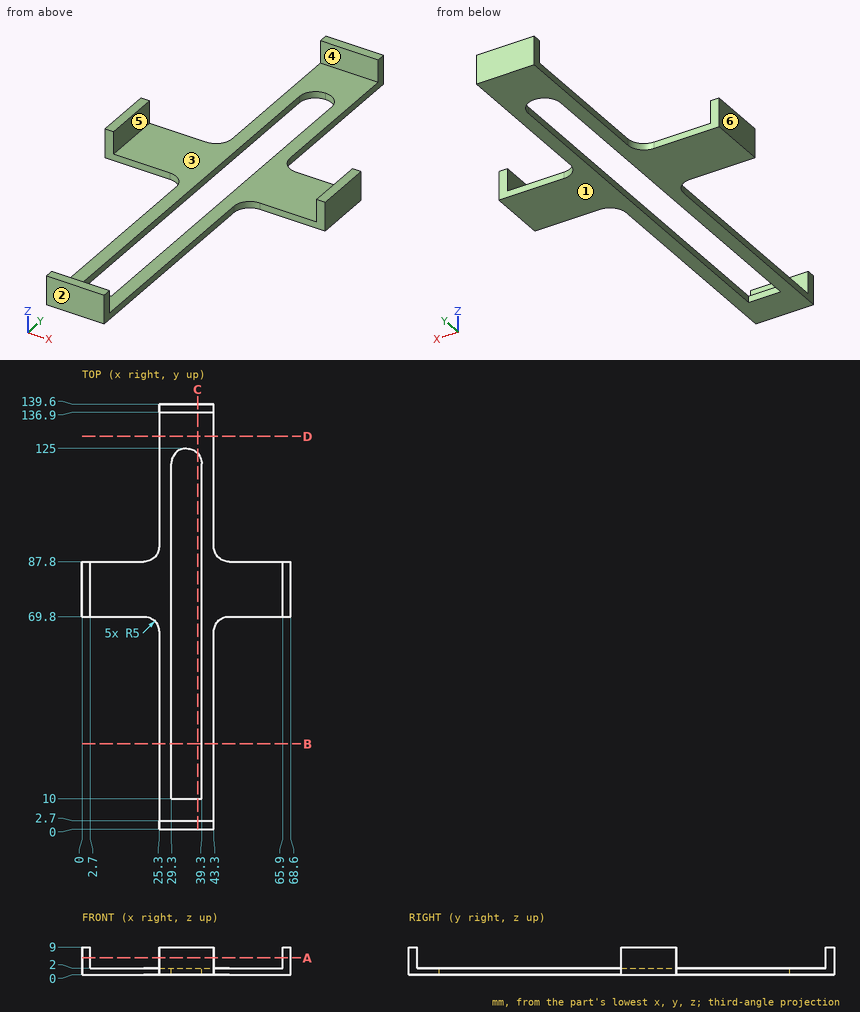
Verification items for this drawing (mm, ordinates from the low corner). A direction names the side the tool comes from. Round coordinates to 2 decimals unless told otherwise and drop trailing zeros. Write each loop counter-clockwise with the first axis right and the second up, starting at its lowest first coordinate (ties: lowest second). Pieces come first, ordered by that corner, then holes. Notation, with made-up numbers: (-8.75, 10) - (20.25, 10) arc R27 ccw to (20.25, 26) - close; hole circle Ø7 at (30.5, 26). An arc over 180 degrees is marked (long way). One line per item, written item: value.
1. Cross-section at C-C on x = 38. Record the boundary of the cut face in (y, z), and give its area (3 significant figures).
The answers:
outline: (0, 0) - (10, 0) - (10, 2) - (2.7, 2) - (2.7, 9) - (0, 9) - close; (123.36, 0) - (139.6, 0) - (139.6, 9) - (136.9, 9) - (136.9, 2) - (123.36, 2) - close
area: 90.3 mm^2
2. Cross-section at A-A on z = 5.5. Record the boundary of the cut face in (x, y).
The answers:
outline: (0, 69.8) - (2.7, 69.8) - (2.7, 87.8) - (0, 87.8) - close; (25.3, 0) - (43.3, 0) - (43.3, 2.7) - (25.3, 2.7) - close; (25.3, 136.9) - (43.3, 136.9) - (43.3, 139.6) - (25.3, 139.6) - close; (65.9, 69.8) - (68.6, 69.8) - (68.6, 87.8) - (65.9, 87.8) - close
3. Cross-section at D-D on y = 129. Record the boundary of the cut face in (x, z), and give its area (3 significant figures).
The answers:
outline: (25.3, 0) - (43.3, 0) - (43.3, 2) - (25.3, 2) - close
area: 36.0 mm^2
4. Depth check by flat-ended pin: pin 1 Ø5 at (x, z) = (50.5, 2) entering from -Y; pin 2 Ø3.5 at (x, z) = (33.5, 4) entering from -Y; pin 3 Ø2 at (y, z) = (64.5, 0.5) entering from -X; pin 4 Ø4 at (y, z) = (97.5, 3.5) entering from +X. Enter the tip coordinate at first touch or a pass-through.
The answers:
pin 1: stops at y = 69.79
pin 2: stops at y = 0
pin 3: stops at x = 25.25
pin 4: stops at x = 43.3
5. Set-up check for the marked faces 5 and 6: record each of +Z, -Z, +X, -X, +Y, -Y from which the full face is reachable in a straight line by a thin tool's end or side.
The answers:
face 5: +Z, +Y, -Y
face 6: +Z, -Z, -X, +Y, -Y
6. Mould release check, pull along Y, two halves, no side actions. Record for the marked faces 1, 2, 3 and 4: released by +Y, released by -Y, zero draft, split by the parting line, or undercut.
The answers:
face 1: zero draft
face 2: released by -Y
face 3: undercut
face 4: undercut
7. Cross-section at B-B on y = 28. Record the boundary of the cut face in (x, z).
The answers:
outline: (25.3, 0) - (29.3, 0) - (29.3, 2) - (25.3, 2) - close; (39.3, 0) - (43.3, 0) - (43.3, 2) - (39.3, 2) - close
8. Scan lines: L1, parallel to Y at x = 27.5, z = 7.5; L2, parallel to X at y = 72, z = 7; L3, parallel to X at y = 46.5, z = 1.5. Record each from-to range of solid material in increasing order.
The answers:
L1: y = 0 to 2.7, 136.9 to 139.6
L2: x = 0 to 2.7, 65.9 to 68.6
L3: x = 25.3 to 29.3, 39.3 to 43.3
